Can you work these out from the model? Positions are in its coordinate system, mm. Face numbers are marked on the shaded views. Round coordinates to 2 decimals unless told otherwise and drop trailing zeros. Write each loop counter-clockwise with the first axis right and the second up, starting at its lowest first coordinate (ties: lowest second). Pieces come first, ordered by that corner, then holes. Notation, with made-up numbers: (-17, 67) -> (28, 67) arc R24 cw to (28, 84) -> close; hole circle Ø7 at (69, -14.75). An arc over 180 degrees is marked (long way). Use CSV: the item, a comma, the result in double quotes.
```python
from build123d import *

# Parameters (mm, degrees)
BOSS_EXTRUDE1_DEPTH         = 4.7625
F_1_4_0_25_DIAMETER_HOLE1_D = 6.35


with BuildPart() as part:
    # Sketch1 → Boss-Extrude1 (new body)
    with BuildSketch(Plane(origin=(0, 0, 0), x_dir=(1, 0, 0), z_dir=(0, 1, 0))):
        with BuildLine():
            Line((-431.938028743, -442.700646237), (-377.110131192, -442.700646237))
            ThreePointArc((-377.110131192, -442.700646237), (-374.763477179, -441.132662155), (-375.314079967, -438.364595013))
            Line((-375.314079967, -438.364595013), (-430.141977519, -383.536697461))
            ThreePointArc((-430.141977519, -383.536697461), (-432.910044661, -382.986094673), (-434.478028743, -385.332748685))
            Line((-434.478028743, -385.332748685), (-434.478028743, -440.160646237))
            ThreePointArc((-434.478028743, -440.160646237), (-433.734079967, -441.956697461), (-431.938028743, -442.700646237))
        make_face()
    extrude(amount=BOSS_EXTRUDE1_DEPTH)

    # 1/4 (0.25) Diameter Hole1 (through all)
    with Locations(Plane(origin=(0, 4.7625, 0), x_dir=(1, 0, 0), z_dir=(0, 1, 0))):
        with Locations((-421.778028743, -404.600646237), (-421.778028743, -430.000646237), (-396.378028743, -430.000646237)):
            Hole(F_1_4_0_25_DIAMETER_HOLE1_D / 2)


solid = part.part
```
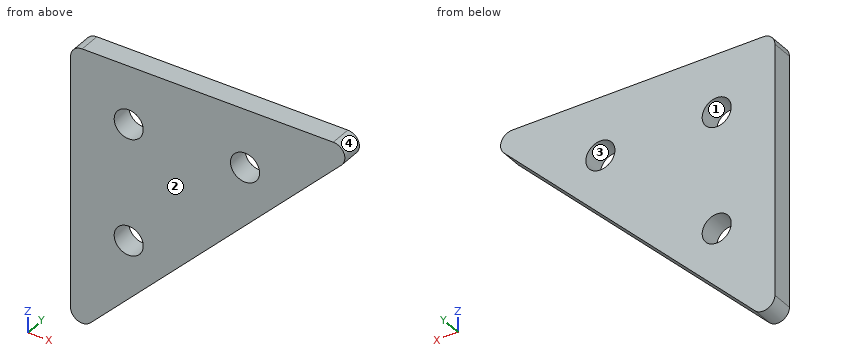
Q1. Will this pin go through, and if not, where does the flat tip stop? P1, Ø4, axis at x = -396.38, z = 430, coming from the +Y side.
Resolved:
P1,"passes through"
Q2. If we mould it in two halves opening along Z, with no side actions, what happens to the marked faces 1, 2, 3 and 4? For each: released by +Z, released by -Z, zero draft, split by the parting line, or undercut.
Resolved:
face 1,"undercut"
face 2,"zero draft"
face 3,"undercut"
face 4,"split by the parting line"
Q3. Suppose I cut it at A-A (x = -423). Write out the boundary of the cut face in (y, z), and give its area (3 significant figures).
Resolved:
outline,"(0, 390.68) -> (4.76, 390.68) -> (4.76, 401.67) -> (0, 401.67) -> close; (0, 407.53) -> (4.76, 407.53) -> (4.76, 427.07) -> (0, 427.07) -> close; (0, 432.93) -> (4.76, 432.93) -> (4.76, 442.7) -> (0, 442.7) -> close"
area,"192 mm^2"
Q4. Please list where these lines run through material, in increasing order: probe 1 along Z at (x, y) = (-396, 3.15); probe 2 along X at (y, z) = (0.7, 402); probe 3 along Z at (x, y) = (-422, 3.2).
Resolved:
probe 1,"z = 417.68 to 426.85, 433.15 to 442.7"
probe 2,"x = -434.48 to -423.6, -419.96 to -411.68"
probe 3,"z = 391.68 to 401.43, 407.77 to 426.83, 433.17 to 442.7"
Q5. Suppose I cut it at C-C (z = 428.5). Write out the boundary of the cut face in (x, y).
Resolved:
outline,"(-434.48, 0) -> (-424.58, 0) -> (-424.58, 4.76) -> (-434.48, 4.76) -> close; (-418.98, 0) -> (-399.18, 0) -> (-399.18, 4.76) -> (-418.98, 4.76) -> close; (-393.58, 0) -> (-385.18, 0) -> (-385.18, 4.76) -> (-393.58, 4.76) -> close"
Q6. Suppose I cut it at B-B (y = 2.45). Write out the boundary of the cut face in (x, z) (3 decimals).
Resolved:
outline,"(-434.478, 385.333) arc R2.54 ccw to (-430.142, 383.537) -> (-375.314, 438.365) arc R2.54 ccw to (-377.11, 442.701) -> (-431.938, 442.701) arc R2.54 ccw to (-434.478, 440.161) -> close; hole circle Ø6.35 at (-421.778, 404.601); hole circle Ø6.35 at (-421.778, 430.001); hole circle Ø6.35 at (-396.378, 430.001)"
Q7. Suppose I cut it at D-D (z = 387.5). Write out the boundary of the cut face in (x, y), and give its area (3 significant figures).
Resolved:
outline,"(-434.48, 0) -> (-426.18, 0) -> (-426.18, 4.76) -> (-434.48, 4.76) -> close"
area,"39.5 mm^2"
